Part model, mm, in its own coordinate system. A direction names the side the tool comes from. Round coordinates to 2 decimals unless told otherwise and drop trailing zeros. Write each loop counter-clockwise with the first axis right and the second up, starting at its lowest first coordinate (ties: lowest second). Pieces come first, ordered by that corner, then holes.
```python
from build123d import *

# Parameters (mm, degrees)
F0_R     = 45
F1_DEPTH = 70
F2_W     = 60
F2_H     = 15
F3_DEPTH = 75
F5_DEPTH = 8
F7_DEPTH = 3


with BuildPart() as f1:
    # F0 (on Front) → F1 (new body)
    with BuildSketch(Plane.XZ):
        Circle(F0_R)
    extrude(amount=F1_DEPTH)

    # F2 (on Front) → F3 (join)
    with BuildSketch(Plane.XZ):
        with Locations((0, 49.5)):
            Rectangle(F2_W, F2_H)
    extrude(amount=F3_DEPTH)

    # F4 (on face) → F5 (cut)
    with BuildSketch(Plane.XY.offset(57)):
        with BuildLine():
            Line((7.5, -28.2193734366), (-7.5, -28.2193734366))
            ThreePointArc((-7.5, -28.2193734366), (0, -35.7193734366), (7.5, -28.2193734366))
        make_face()
        with BuildLine():
            ThreePointArc((7.5, -28.2193734366), (0, -20.7193734366), (-7.5, -28.2193734366))
            Line((-7.5, -28.2193734366), (7.5, -28.2193734366))
        make_face()
        with BuildLine():
            Line((7.5, -10.2193734366), (-7.5, -10.2193734366))
            ThreePointArc((-7.5, -10.2193734366), (0, -17.7193734366), (7.5, -10.2193734366))
        make_face()
        with BuildLine():
            Line((8.5, -46.1915741923), (-6.5, -46.1915741923))
            ThreePointArc((-6.5, -46.1915741923), (1, -53.6915741923), (8.5, -46.1915741923))
        make_face()
        with BuildLine():
            ThreePointArc((8.5, -64.1915741923), (1, -56.6915741923), (-6.5, -64.1915741923))
            Line((-6.5, -64.1915741923), (8.5, -64.1915741923))
        make_face()
        with BuildLine():
            Line((8.5, -64.1915741923), (-6.5, -64.1915741923))
            ThreePointArc((-6.5, -64.1915741923), (1, -71.6915741923), (8.5, -64.1915741923))
        make_face()
        with BuildLine():
            ThreePointArc((8.5, -46.1915741923), (1, -38.6915741923), (-6.5, -46.1915741923))
            Line((-6.5, -46.1915741923), (8.5, -46.1915741923))
        make_face()
        with BuildLine():
            ThreePointArc((7.5, -10.2193734366), (0, -2.7193734366), (-7.5, -10.2193734366))
            Line((-7.5, -10.2193734366), (7.5, -10.2193734366))
        make_face()
        with BuildLine():
            ThreePointArc((7.5, -10.2193734366), (0, -17.7193734366), (-7.5, -10.2193734366))
            Line((-7.5, -10.2193734366), (-7.5, -28.2193734366))
            ThreePointArc((-7.5, -28.2193734366), (0, -20.7193734366), (7.5, -28.2193734366))
            Line((7.5, -28.2193734366), (7.5, -10.2193734366))
        make_face()
        with BuildLine():
            ThreePointArc((8.5, -46.1915741923), (1, -53.6915741923), (-6.5, -46.1915741923))
            Line((-6.5, -46.1915741923), (-6.5, -64.1915741923))
            ThreePointArc((-6.5, -64.1915741923), (1, -56.6915741923), (8.5, -64.1915741923))
            Line((8.5, -64.1915741923), (8.5, -46.1915741923))
        make_face()
    extrude(amount=-F5_DEPTH, mode=Mode.SUBTRACT)

    # F6 (on face) → F7 (join)
    with BuildSketch(Plane.XY.offset(57)):
        with BuildLine():
            Line((-7.5, -10.2193734366), (-7.5, -28.2193734366))
            Line((-7.5, -28.2193734366), (-4.3874821937, -13.5458519471))
            Line((-4.3874821937, -13.5458519471), (-4.5479531951, -4.2556395614))
            ThreePointArc((-4.5479531951, -4.2556395614), (-6.7215938944, -6.8921861082), (-7.5, -10.2193734366))
        make_face()
        with BuildLine():
            Line((4.3874821937, -13.5458519471), (7.5, -28.2193734366))
            Line((7.5, -28.2193734366), (7.5, -10.2193734366))
            ThreePointArc((7.5, -10.2193734366), (6.67668018, -6.802951072), (4.3874821937, -4.1366109064))
            Line((4.3874821937, -4.1366109064), (4.3874821937, -13.5458519471))
        make_face()
        with BuildLine():
            Line((5.5, -49.4946357356), (8.5, -64.1915741923))
            Line((8.5, -64.1915741923), (8.5, -46.1915741923))
            ThreePointArc((8.5, -46.1915741923), (7.7082039325, -42.837472226), (5.5, -40.1915741923))
            Line((5.5, -40.1915741923), (5.5, -49.4946357356))
        make_face()
        with BuildLine():
            Line((-6.5, -46.1915741923), (-6.5, -64.1915741923))
            Line((-6.5, -64.1915741923), (-3.5, -49.4946357356))
            Line((-3.5, -49.4946357356), (-3.5, -40.1915741923))
            ThreePointArc((-3.5, -40.1915741923), (-5.7082039325, -42.837472226), (-6.5, -46.1915741923))
        make_face()
    extrude(amount=-F7_DEPTH)


solid = f1.part
```
Q1. Cut at C-C on x = 0. Write the cut outline in (y, z).
Values follow:
outline: (-75, 42) - (-70, 42) - (-70, -45) - (0, -45) - (0, 57) - (-2.72, 57) - (-2.72, 49) - (-35.72, 49) - (-35.72, 57) - (-38.76, 57) - (-38.76, 49) - (-71.62, 49) - (-71.62, 57) - (-75, 57) - close
Q2. Which spindle directions (+Z, -Z, +X, -X, +Y, -Y) get a long thin tool onto all of the face, cutting with end or side? Do faces 1 (the flat face through (30, -37, 49)), 2 (the cylindrical face through (0.16, -2.72, 52.17)), 3 (the flat face through (-5.966, -20.985, 55.521)). Say none if no direction does.
Values follow:
face 1: +Z, +X, +Y, -Y
face 2: none
face 3: +Z
Q3. Cut at D-D on z = 0. Write the cut outline in (x, y), plus the area to 3 significant figures.
Values follow:
outline: (-45, -70) - (45, -70) - (45, 0) - (-45, 0) - close
area: 6,300 mm2
Q4. Drop flat-ended pins along their axis: pin 1 (1.5 mm diameter, centred on y = -22.5, z = 52.5, fed in from -X); pin 2 (1.5 mm diameter, centred on x = -9.5, z = -10, fed in from +Y); pin 3 (7.5 mm diameter, centred on x = 3, y = -60.5, fed in from +Z); pin 4 (7.5 mm diameter, centred on y = -48.5, z = 53, fed in from +X). Give the stop position or say it passes through.
Values follow:
pin 1: stops at x = -30
pin 2: stops at y = 0
pin 3: stops at z = 49
pin 4: stops at x = 30
Q5. Cut at B-B on y = -17.5. Write the cut outline in (x, z), plus the area to 3 significant figures.
Values follow:
outline: (-30, 42) - (-16.16, 42) arc R45 ccw (long way) to (16.16, 42) - (30, 42) - (30, 57) - (5.23, 57) - (5.23, 54) - (7.5, 54) - (7.5, 49) - (-7.5, 49) - (-7.5, 54) - (-5.23, 54) - (-5.23, 57) - (-30, 57) - close
area: 7,090 mm2
Q6. Mould opens along X. For faces 4 (the flat face through (-30, -37, 49)), 5 (the flat face through (-1, 0, 7)), 6 (the cylindrical face through (1.165, -38.693, 52.167)), 7 (the flat face through (-7.5, -19, 52)) say: +X half, -X half, draft (parallel to the pull), parting line (faces both ways), or undercut.
Values follow:
face 4: -X half
face 5: draft
face 6: undercut
face 7: undercut
Q7. Cut at A-A on x = 22.5. Write the cut outline in (y, z), plus the area to 3 significant figures.
Values follow:
outline: (-75, 42) - (0, 42) - (0, 57) - (-75, 57) - close; (-70, -38.97) - (0, -38.97) - (0, 38.97) - (-70, 38.97) - close
area: 6,580 mm2
Q8. Wall check: L1, parallel to Z at x = -18.5, y = -31.5; L2, parallel to Z at x = 22, y = -25; L3, parallel to Z at x = 17.5, y = -70.5. Give the ranges that are in metal, low to high.
Values follow:
L1: z = -41.02 to 41.02, 42 to 57
L2: z = -39.26 to 39.26, 42 to 57
L3: z = 42 to 57
